Read the model definition and answer for the solid it produces. Units are mm, in the model's axes. A direction names the side the tool comes from. Round coordinates to 2 decimals unless told otherwise and drop trailing zeros. Order: outer loops, then holes, each group sorted by start corner. A loop starts at its lowest first (then second) coordinate and runs counter-clockwise, first axis right, second up. Notation, with made-up numbers: (52, -29) - (84, -29) arc R28 cw to (84, -4) - close; hole circle Ø3 at (-7, -19.75). An arc over 180 degrees is marked (long way). Put each result on its own line as item: value. Start each with the question number.
Q1. Section A-A on z = 5 is taken. Give the vertices of the cut face in (x, y).
Q2. Section C-C on y = 2.75 is taken. Give the vertices of the cut face in (x, z), then the cut area to 3 significant figures.
Q3. This flat-tipped pin is pushed along its axis until it touches: pin 1 Ø1.1 at (x, y) = (-0.5, 5.5) entering from -Z. Where does it stop, or does it pass through?
Q4. Section B-B on y = -2 is taken. Give the vertices of the cut face in (x, z), then the cut area to 3 significant figures.
Q5. Find the intervals of material crossed by line 1 along Y through (x, z) = (0, 24.2); line 2 along Y through (x, z) = (0, 24.1); line 3 along Z through (x, y) = (2.25, -4.25), in increasing order. Write a range as from..to.
Q6. For a pull along X with two mould halves and no side action, classify faces 4 (the face through (-12.5, 0, 12)), 5 (the face through (0, 12.5, 12)), 6 (the face through (12.5, 0, 12)), 7 (the face through (0, 0, 10)) as pulls with the +X half, pulls with the -X half, needs draft (parallel to the pull), parting line crosses it, or undercut.
Q7. Which of the six approach directions +Z, -Z, +X, -X, +Y, -Y give full straight-line access (tool end or side, diameter ignored) to faces 1 (the face through (0, 5, 10)), 2 (the face through (-11.9, -0.2, 24.4)), 3 (the face through (0, 0, 23))?
from build123d import *

# Parameters (mm, degrees)
F0_W     = 25
F0_H     = 25
F1_DEPTH = 25
F2_R     = 6
F3_DEPTH = 2
F5_DEPTH = 10
F6_SIZE  = 1.2


with BuildPart() as f1:
    # F0 (on Top) → F1 (new body)
    with BuildSketch(Plane.XY):
        Rectangle(F0_W, F0_H)
    extrude(amount=F1_DEPTH)

    # F2 (on face) → F3 (cut)
    with BuildSketch(Plane.XY.offset(25)):
        Circle(F2_R)
    extrude(amount=-F3_DEPTH, mode=Mode.SUBTRACT)

    # F4 (on face) → F5 (cut)
    with BuildSketch(Plane(origin=(0, 0, 0), x_dir=(1, 0, 0), z_dir=(0, 0, -1))):
        with BuildLine():
            ThreePointArc((0, -3.75), (-1.75, -5.5), (0, -7.25))
            Line((0, -7.25), (0, -3.75))
        make_face()
        with BuildLine():
            ThreePointArc((0, 7.25), (-1.75, 5.5), (0, 3.75))
            Line((0, 3.75), (0, 7.25))
        make_face()
        with BuildLine():
            Line((0, 7.25), (0, 3.75))
            ThreePointArc((0, 3.75), (1.237437, 4.262563), (1.75, 5.5))
            ThreePointArc((1.75, 5.5), (1.237437, 6.737437), (0, 7.25))
        make_face()
        with BuildLine():
            ThreePointArc((0, 1.5), (-1.5, 0), (0, -1.5))
            Line((0, -1.5), (0, 1.5))
        make_face()
        with BuildLine():
            Line((0, 1.5), (0, -1.5))
            ThreePointArc((0, -1.5), (1.06066, -1.06066), (1.5, 0))
            ThreePointArc((1.5, 0), (1.06066, 1.06066), (0, 1.5))
        make_face()
        with BuildLine():
            Line((0, -3.75), (0, -7.25))
            ThreePointArc((0, -7.25), (1.237437, -6.737437), (1.75, -5.5))
            ThreePointArc((1.75, -5.5), (1.237437, -4.262563), (0, -3.75))
        make_face()
    extrude(amount=-F5_DEPTH, mode=Mode.SUBTRACT)

    # F6
    f6_edges = [f1.edges().sort_by_distance(p)[0] for p in [
        (0, 12.5, 25),
        (-12.5, 0, 25),
        (0, -12.5, 25),
        (12.5, 0, 25),
    ]]
    chamfer(f6_edges, length=F6_SIZE)


solid = f1.part
Findings:
1. outline: (-12.5, -12.5) - (12.5, -12.5) - (12.5, 12.5) - (-12.5, 12.5) - close; hole circle Ø3.5 at (0, -5.5); hole circle Ø3.5 at (0, 5.5); hole circle Ø3 at (0, 0)
2. outline: (-12.5, 0) - (12.5, 0) - (12.5, 23.8) - (11.3, 25) - (5.33, 25) - (5.33, 23) - (-5.33, 23) - (-5.33, 25) - (-11.3, 25) - (-12.5, 23.8) - close
2. area: 602 mm2
3. pin 1: z = 10
4. outline: (-12.5, 0) - (12.5, 0) - (12.5, 23.8) - (11.3, 25) - (5.66, 25) - (5.66, 23) - (-5.66, 23) - (-5.66, 25) - (-11.3, 25) - (-12.5, 23.8) - close
4. area: 601 mm2
5. line 1: -12.1..-6, 6..12.1
5. line 2: -12.2..-6, 6..12.2
5. line 3: 0..23
6. face 4: pulls with the -X half
6. face 5: needs draft
6. face 6: pulls with the +X half
6. face 7: undercut
7. face 1: -Z
7. face 2: +Z, -X, +Y, -Y
7. face 3: +Z
